```python
from build123d import *

# Parameters (mm, degrees)
SKETCH1_W                      = 28
SKETCH1_H                      = 28
BOSS_EXTRUDE1_DEPTH            = 3
SKETCH2_R                      = 8.75
CUT_EXTRUDE1_DEPTH             = 21.024984395
M3_CLEARANCE_HOLE1_D           = 3.4
M3_CLEARANCE_HOLE1_CSINK_D     = 3.45
M3_CLEARANCE_HOLE1_CSINK_ANGLE = 90
FILLET1_R                      = 3


with BuildPart() as part:
    # Sketch1 → Boss-Extrude1 (new body)
    with BuildSketch(Plane(origin=(0, 0, 0), x_dir=(1, 0, 0), z_dir=(0, 1, 0))):
        Rectangle(SKETCH1_W, SKETCH1_H)
    extrude(amount=BOSS_EXTRUDE1_DEPTH)

    # Sketch2 → Cut-Extrude1 (cut, through all)
    with BuildSketch(Plane(origin=(0, 3, 0), x_dir=(1, 0, 0), z_dir=(0, 1, 0))):
        with Locations(Location((0, 0, 0), (0, 0, 270))):
            Circle(SKETCH2_R)
    extrude(amount=-CUT_EXTRUDE1_DEPTH, mode=Mode.SUBTRACT)

    # M3 Clearance Hole1 (through all)
    with Locations(Plane(origin=(0, 3, 0), x_dir=(1, 0, 0), z_dir=(0, 1, 0))):
        with Locations((-9.545941546, 9.545941546), (9.545941546, 9.545941546), (9.545941546, -9.545941546), (-9.545941546, -9.545941546)):
            CounterSinkHole(M3_CLEARANCE_HOLE1_D / 2, M3_CLEARANCE_HOLE1_CSINK_D / 2, counter_sink_angle=M3_CLEARANCE_HOLE1_CSINK_ANGLE)

    # Fillet1
    fillet1_edges = [part.edges().sort_by_distance(p)[0] for p in [
        (-14, 1.5, -14),
        (14, 1.5, -14),
        (14, 1.5, 14),
        (-14, 1.5, 14),
    ]]
    fillet(fillet1_edges, radius=FILLET1_R)


solid = part.part
```
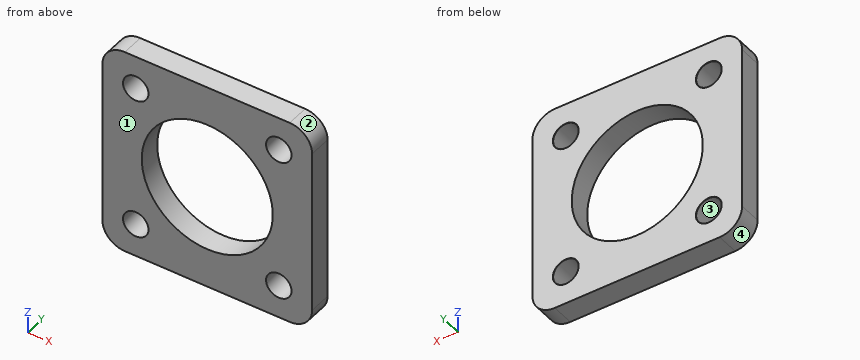
Check sheet for the modelled part. Datum: model origin and axes. Units: mm. Face numbers are marked on the shaded views. Round coordinates to 2 decimals unless told otherwise and drop trailing zeros. Loops run counter-clockwise (first coordinate to the right, second up) from the corner with the lowest first, then second, coordinate; pieces in that order, holes last. Notation, with made-up numbers: (33.25, 8.25) -> (78.25, 8.25) arc R17 cw to (78.25, 41.25) -> close; hole circle Ø11 at (-22, 2). An arc over 180 degrees is marked (long way). Answer in a Markdown table with one row per item.
Q1. Sectioned sample at A-A on z = 0. Enter the section's corners in (x, y), then the cut area to 3 significant figures.
Data:
| item | result |
|---|---|
| outline | (-14, 0) -> (-8.75, 0) -> (-8.75, 3) -> (-14, 3) -> close; (8.75, 0) -> (14, 0) -> (14, 3) -> (8.75, 3) -> close |
| area | 31.5 mm^2 |
Q2. Release check for a two-part mould opening along X. For the marked faces 1, 2, 3 and 4 record: released by +X, released by -X, zero draft, split by the parting line, or undercut.
Data:
| item | result |
|---|---|
| face 1 | zero draft |
| face 2 | released by +X |
| face 3 | undercut |
| face 4 | released by -X |
Q3. Sectioned sample at C-C on y = 2.15. Enter the section's corners in (x, z), then the cut area to 3 significant figures.
Data:
| item | result |
|---|---|
| outline | (-14, -11) arc R3 ccw to (-11, -14) -> (11, -14) arc R3 ccw to (14, -11) -> (14, 11) arc R3 ccw to (11, 14) -> (-11, 14) arc R3 ccw to (-14, 11) -> close; hole circle Ø3.4 at (-9.55, -9.55); hole circle Ø3.4 at (-9.55, 9.55); hole circle Ø17.5 at (0, 0); hole circle Ø3.4 at (9.55, -9.55); hole circle Ø3.4 at (9.55, 9.55) |
| area | 499 mm^2 |
Q4. Thickness scan on L1, parallel to Z at x = -9, y = 2.15; L2, parallel to Z at x = 7.75, y = 2; L3, parallel to X at y = 0.9, z = -0.5. Record the ranges inside material, lowest first.
Data:
| item | result |
|---|---|
| L1 | z = -14 to -11.16, -7.94 to 7.94, 11.16 to 14 |
| L2 | z = -14 to -4.06, 4.06 to 14 |
| L3 | x = -14 to -8.74, 8.74 to 14 |
Q5. Go/stop test with a flat-tipped pin: P1, Ø10.5, axis at x = 0, z = 0, coming from the -Y side. Record where the tip stops, or that it passes through.
Data:
| item | result |
|---|---|
| P1 | passes through |
Q6. Sectioned sample at B-B on x = 0. Enter the section's corners in (y, z), then the cut area to 3 significant figures.
Data:
| item | result |
|---|---|
| outline | (0, -14) -> (3, -14) -> (3, -8.75) -> (0, -8.75) -> close; (0, 8.75) -> (3, 8.75) -> (3, 14) -> (0, 14) -> close |
| area | 31.5 mm^2 |
